Part model, mm, in its own coordinate system. Round coordinates to 2 decimals unless told otherwise and drop trailing zeros. Loops run counter-clockwise (first coordinate to the right, second up) from the corner with the lowest first, then second, coordinate; pieces in that order, holes last. Notation, with made-up numbers: (4.25, -24.5) - (25.25, -24.5) arc R21 cw to (25.25, 1.5) - close; hole circle Ø11 at (26, -25). An arc over 180 degrees is marked (long way). Write each question's results on one line, items separated by ' | '. Start each with the question number.
(1) Cut at C-C, the plane x = 8. List the corners of the cut face in (y, z).
(2) Drill centre lines: L1, parallel to X at y = -6.5, z = 1.45; L2, parallel to Y at x = 65.5, z = 1.35; L3, parallel to X at y = -57, z = 0.35. Where is each one in solid material? Low to high.
(3) Cut at D-D, the plane x = 40. List the corners of the cut face in (y, z).
(4) Cut at B-B, the plane z = 0.75. List the corners of the cut face in (x, y), then the cut area to 3 significant figures.
(5) Cut at A-A, the plane y = -8. List the corners of the cut face in (x, z).
(6) Flat gauge pin, fed straight in: P1, Ø0.8, axis at y = -35, z = 0.5, coming from the +X side. Where does the tip first touch, or does it go through?
from build123d import *

# Parameters (mm, degrees)
SKETCH1_W           = 80
SKETCH1_H           = 80
BOSS_EXTRUDE1_DEPTH = 1.5
SKETCH2_W           = 64
SKETCH2_H           = 64
CUT_EXTRUDE1_DEPTH  = 2.5
HOLE1_AT_2_COUNT    = 2
HOLE1_AT_2_PITCH    = 32
HOLE1_AT_3_COUNT    = 2
HOLE1_AT_3_PITCH    = 64
HOLE1_AT_4_COUNT    = 2
HOLE1_AT_4_PITCH    = 32
HOLE1_AT_5_COUNT    = 2
HOLE1_AT_5_PITCH    = 64


with BuildPart() as part:
    # Sketch1 → Boss-Extrude1 (new body)
    with BuildSketch(Plane.XY.offset(1.5)):
        with Locations((40, -40)):
            Rectangle(SKETCH1_W, SKETCH1_H)
    extrude(amount=-BOSS_EXTRUDE1_DEPTH)

    # Sketch2 → Cut-Extrude1 (cut, through all)
    with BuildSketch(Plane(origin=(0, 0, 0), x_dir=(-1, 0, 0), z_dir=(0, 0, -1))):
        with Locations((-48, -48)):
            Rectangle(SKETCH2_W, SKETCH2_H)
    extrude(amount=-CUT_EXTRUDE1_DEPTH, mode=Mode.SUBTRACT)

    # Sketch3 → Hole1 (revolve, cut)
    with BuildSketch(Plane(origin=(8, -8, 1.5), x_dir=(0, -1, 0), z_dir=(1, 0, 0))):
        Polygon((0, 0), (0, 1.5), (2.25, 1.5), (3.75, 0), align=None)
    hole1 = revolve(axis=Axis((8, -8, -108.5), (0, 0, 1)), mode=Mode.SUBTRACT)

    # Hole1 at 2: Hole1 ×2
    with Locations(*[(i * HOLE1_AT_2_PITCH, 0, 0) for i in range(1, HOLE1_AT_2_COUNT)]):
        add(hole1, mode=Mode.SUBTRACT)

    # Hole1 at 3: Hole1 ×2
    with Locations(*[(i * HOLE1_AT_3_PITCH, 0, 0) for i in range(1, HOLE1_AT_3_COUNT)]):
        add(hole1, mode=Mode.SUBTRACT)

    # Hole1 at 4: Hole1 ×2
    with Locations(*[(0, -i * HOLE1_AT_4_PITCH, 0) for i in range(1, HOLE1_AT_4_COUNT)]):
        add(hole1, mode=Mode.SUBTRACT)

    # Hole1 at 5: Hole1 ×2
    with Locations(*[(0, -i * HOLE1_AT_5_PITCH, 0) for i in range(1, HOLE1_AT_5_COUNT)]):
        add(hole1, mode=Mode.SUBTRACT)


solid = part.part
A:
1) outline: (-80, 0) - (-74.25, 0) - (-75.75, 1.5) - (-80, 1.5) - close; (-69.75, 0) - (-42.25, 0) - (-43.75, 1.5) - (-68.25, 1.5) - close; (-37.75, 0) - (-10.25, 0) - (-11.75, 1.5) - (-36.25, 1.5) - close; (-5.75, 0) - (0, 0) - (0, 1.5) - (-4.25, 1.5) - close
2) L1: 0 to 4.62, 11.38 to 36.62, 43.38 to 68.62, 75.38 to 80 | L2: -16 to 0 | L3: 0 to 16
3) outline: (-16, 0) - (-10.25, 0) - (-11.75, 1.5) - (-16, 1.5) - close; (-5.75, 0) - (0, 0) - (0, 1.5) - (-4.25, 1.5) - close
4) outline: (0, -80) - (16, -80) - (16, -16) - (80, -16) - (80, 0) - (0, 0) - close; hole circle Ø6 at (8, -72); hole circle Ø6 at (8, -40); hole circle Ø6 at (8, -8); hole circle Ø6 at (40, -8); hole circle Ø6 at (72, -8) | area: 2,160 mm2
5) outline: (0, 0) - (5.75, 0) - (4.25, 1.5) - (0, 1.5) - close; (10.25, 0) - (37.75, 0) - (36.25, 1.5) - (11.75, 1.5) - close; (42.25, 0) - (69.75, 0) - (68.25, 1.5) - (43.75, 1.5) - close; (74.25, 0) - (80, 0) - (80, 1.5) - (75.75, 1.5) - close
6) P1: x = 16
